Input: part model. Units: mm. Frame: model coordinates. Round coordinates to 2 decimals unless told otherwise and drop trailing zeros. Loops run counter-clockwise (first coordinate to the right, second up) from the corner with the lowest first, then second, coordinate; pieces in that order, holes last. Notation, with made-up numbers: (-9.75, 8) -> (30.25, 8) arc R24 cw to (30.25, 33) -> close; hole circle Ø4 at (47, 33). An arc over 180 degrees is marked (long way). Answer as a JSON object with one key per item and string values.
```python
from build123d import *

# Parameters (mm, degrees)
BOSS_EXTRUDE1_DEPTH = 6.35
SKETCH2_W           = 6.35
SKETCH2_H           = 19.05
SKETCH2_W_2         = 12.7
SKETCH2_H_2         = 6.35
SKETCH2_R           = 1.778
CUT_EXTRUDE1_DEPTH  = 127.683693603


with BuildPart() as part:
    # Sketch1 → Boss-Extrude1 (new body)
    with BuildSketch(Plane.XY):
        Polygon((-46.99, 111.125), (-38.1, 111.125), (-38.1, 117.475), (-12.7, 117.475), (-12.7, 111.125), (12.7, 111.125), (12.7, 117.475), (38.1, 117.475), (38.1, 111.125), (46.99, 111.125), (46.99, -111.125), (38.1, -111.125), (38.1, -117.475), (12.7, -117.475), (12.7, -111.125), (-12.7, -111.125), (-12.7, -117.475), (-38.1, -117.475), (-38.1, -111.125), (-46.99, -111.125), align=None)
    extrude(amount=BOSS_EXTRUDE1_DEPTH)

    # Sketch2 → Cut-Extrude1 (cut, through all)
    with BuildSketch(Plane(origin=(0, 0, 0), x_dir=(-1, 0, 0), z_dir=(0, 0, -1))):
        with Locations((-43.815, -54.2076454)):
            Rectangle(SKETCH2_W, SKETCH2_H)
        with Locations((-43.815, -16.1076454)):
            Rectangle(SKETCH2_W, SKETCH2_H)
        with Locations((-34.13125, -79.6076454)):
            Rectangle(SKETCH2_W_2, SKETCH2_H_2)
        with Locations((25.4, -15.485506714)):
            Rectangle(SKETCH2_W_2, SKETCH2_H_2)
        with Locations((25.4, -44.695506714)):
            Rectangle(SKETCH2_W_2, SKETCH2_H_2)
        with Locations((-18.25625, -42.753213284)):
            Circle(SKETCH2_R)
    extrude(amount=-CUT_EXTRUDE1_DEPTH, mode=Mode.SUBTRACT)


solid = part.part
```
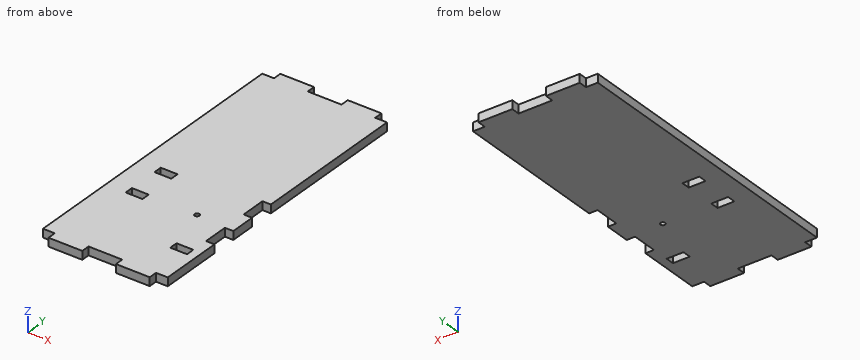
1) Section B-B, the plane x = 34.5. Output: boundary loops of the cut face in (y, z) (3 decimals).
Output:
{"outline": "(-117.475, 0) -> (-82.783, 0) -> (-82.783, 6.35) -> (-117.475, 6.35) -> close; (-76.433, 0) -> (117.475, 0) -> (117.475, 6.35) -> (-76.433, 6.35) -> close"}
2) Ray query, probe 1 along Y at (x, z) = (-22, 3) (1 decimal); probe 2 along Y at (x, z) = (39, 1.5) (3 decimals); probe 3 along Y at (x, z) = (41.5, 1.5) (3 decimals). Return the intervals inside material, ascending.
Output:
{"probe 1": "y = -117.5 to -47.9, -41.5 to -18.7, -12.3 to 117.5", "probe 2": "y = -111.125 to -82.783, -76.433 to 111.125", "probe 3": "y = -111.125 to -63.733, -44.683 to -25.633, -6.583 to 111.125"}
3) Contact query for flat-ended pins moving along their axis: P1, Ø3, axis at y = 115.5, z = 2.5, coming from the +X side; P2, Ø12, axis at x = 5, y = 33, coming from the -Z side; P3, Ø3, axis at x = 41.5, z = 3.5, coming from the -Y side (3 decimals); P4, Ø1.9, axis at y = -54, z = 3, coming from the +X side. Output: stop coordinate, or through.
Output:
{"P1": "stops at x = 38.1", "P2": "stops at z = 0", "P3": "stops at y = -111.125", "P4": "stops at x = 40.64"}
4) Section A-A, the plane x = -29. Count the separate pieces of the cut face and the enclosed holes in it, plus the area to 3 significant figures.
Output:
{"separate pieces": "3", "enclosed holes": "0", "area": "1,410 mm^2"}
5) Section C-C, the plane x = 4. Output: boundary loops of the cut face in (y, z) (3 decimals), plus the area to 3 significant figures.
Output:
{"outline": "(-111.125, 0) -> (111.125, 0) -> (111.125, 6.35) -> (-111.125, 6.35) -> close", "area": "1,410 mm^2"}
